Build history of the part. All positions in model axes, mm. Give positions to 0.01 mm unless a question says otherwise; leave off trailing zeros. Loops run counter-clockwise (first coordinate to the right, second up) from the corner with the lowest first, then second, coordinate; pieces in that order, holes last. Notation, with made-up numbers: (41.25, 75) -> (60.25, 75) arc R21 cw to (60.25, 103) -> close; hole circle Ø9 at (47.25, 71). An arc over 180 degrees is marked (long way). Answer as a JSON object with one key per item and string values. Group by question number.
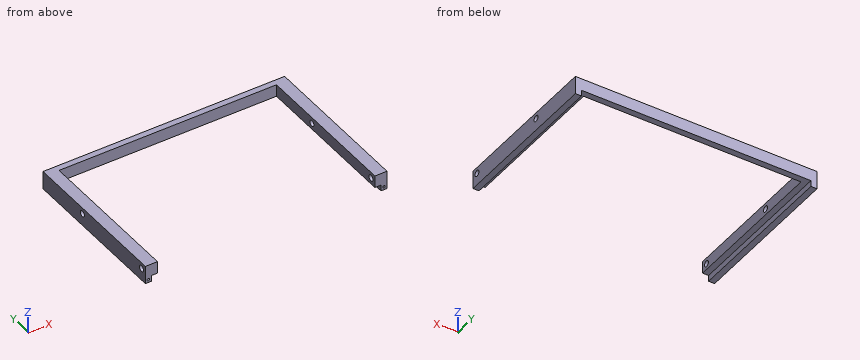
from build123d import *

# Parameters (mm, degrees)
F0_W      = 1300
F0_H      = 150
F1_DEPTH  = 50
F2_W      = 1300
F2_H      = 100
F3_DEPTH  = 50
F4_W      = 50
F4_H      = 100
F5_DEPTH  = 1800
F6_DEPTH  = 100
F7_W      = 100
F7_H      = 100
F8_DEPTH  = 1250
F9_W      = 50
F9_H      = 1300
F10_DEPTH = 50
F11_R     = 25
F12_DEPTH = 200
F13_R     = 25
F14_DEPTH = 200
F15_R     = 10
F16_DEPTH = 25
F17_R     = 10
F18_DEPTH = 25


with BuildPart() as f1:
    # F0 (on Right) → F1 (new body)
    with BuildSketch(Plane.YZ):
        Rectangle(F0_W, F0_H)
    extrude(amount=F1_DEPTH)

    # F2 (on face) → F3 (join)
    with BuildSketch(Plane.YZ.offset(50)):
        with Locations((0, 25)):
            Rectangle(F2_W, F2_H)
    extrude(amount=F3_DEPTH)

    # F4 (on face) → F5 (join)
    with BuildSketch(Plane.YZ.offset(100)):
        with Locations((625, 25)):
            Rectangle(F4_W, F4_H)
    extrude(amount=F5_DEPTH)

    # F6 (add): a face of the model
    f6_faces = [f1.faces().sort_by_distance(p)[0] for p in [
        (1900, 625, 25),
    ]]
    extrude(f6_faces, amount=F6_DEPTH)

    # F7 (on face) → F8 (join)
    with BuildSketch(Plane.XZ.offset(-600)):
        with Locations((1950, 25)):
            Rectangle(F7_W, F7_H)
    extrude(amount=F8_DEPTH)

    # F9 (on face) → F10 (join)
    with BuildSketch(Plane(origin=(0, 0, -25), x_dir=(1, 0, 0), z_dir=(0, 0, -1))):
        with Locations((1975, 0)):
            Rectangle(F9_W, F9_H)
    extrude(amount=F10_DEPTH)

    # F11 (on face) → F12 (cut)
    with BuildSketch(Plane.YZ.offset(100)):
        with Locations((150, 25)):
            Circle(F11_R)
        with Locations((-600, 25)):
            Circle(F11_R)
    extrude(amount=-F12_DEPTH, mode=Mode.SUBTRACT)

    # F13 (on face) → F14 (cut)
    with BuildSketch(Plane(origin=(1900, 0, 0), x_dir=(0, -1, 0), z_dir=(-1, 0, 0))):
        with Locations((-150, 25)):
            Circle(F13_R)
        with Locations((600, 25)):
            Circle(F13_R)
    extrude(amount=-F14_DEPTH, mode=Mode.SUBTRACT)

    # F15 (on face) → F16 (cut)
    with BuildSketch(Plane.XZ.offset(650)):
        with Locations((25, -50)):
            Circle(F15_R)
    extrude(amount=-F16_DEPTH, mode=Mode.SUBTRACT)

    # F17 (on face) → F18 (cut)
    with BuildSketch(Plane.XZ.offset(650)):
        with Locations((1975, -50)):
            Circle(F17_R)
    extrude(amount=-F18_DEPTH, mode=Mode.SUBTRACT)


solid = f1.part
(1) Saw through at C-C on z = 25. List the corners of the cut face in (x, y).
(2) Saw through at A-A on y = 258. List the corners of the cut face in (x, z).
(3) Pin check, flat tips, straight feed: pin 1 (16 mm diameter, centred on x = 25, z = -50, fed in from -Y); pin 2 (3 mm diameter, centred on x = 1384.5, z = -8, fed in from -Y). Stop position of each tip, or through.
(4) Probe line 1 along X through (y, z) = (509, 15.5); line 2 along X through (y, z) = (513, -61); line 3 along Z through (x, y) = (22, 150). List the from-to ranges inside material, lowest first. Write a range as [from, to].
(5) Saw through at B-B on y = -600. List the corners of the cut face in (x, z), plus the area to 3 significant figures.
(6) Saw through at D-D on x = 607. List the corners of the cut face in (y, z), plus the area to 3 significant figures.
Calculated:
{
 "1": {"outline": "(0, -650) -> (100, -650) -> (100, -625) -> (0, -625) -> close; (0, -575) -> (100, -575) -> (100, 125) -> (0, 125) -> close; (0, 175) -> (100, 175) -> (100, 600) -> (1900, 600) -> (1900, 175) -> (2000, 175) -> (2000, 650) -> (0, 650) -> close; (1900, -650) -> (2000, -650) -> (2000, -625) -> (1900, -625) -> close; (1900, -575) -> (2000, -575) -> (2000, 125) -> (1900, 125) -> close"},
 "2": {"outline": "(0, -75) -> (50, -75) -> (50, -25) -> (100, -25) -> (100, 75) -> (0, 75) -> close; (1900, -25) -> (1950, -25) -> (1950, -75) -> (2000, -75) -> (2000, 75) -> (1900, 75) -> close"},
 "3": {"pin 1": "stops at y = -625", "pin 2": "stops at y = 600"},
 "4": {"line 1": "x = [0, 100], [1900, 2000]", "line 2": "x = [0, 50], [1950, 2000]", "line 3": "z = [-75, 0], [50, 75]"},
 "5": {"outline": "(0, -75) -> (50, -75) -> (50, -25) -> (100, -25) -> (100, 0) -> (0, 0) -> close; (0, 50) -> (100, 50) -> (100, 75) -> (0, 75) -> close; (1900, -25) -> (1950, -25) -> (1950, -75) -> (2000, -75) -> (2000, 0) -> (1900, 0) -> close; (1900, 50) -> (2000, 50) -> (2000, 75) -> (1900, 75) -> close", "area": "15,000 mm^2"},
 "6": {"outline": "(600, -25) -> (650, -25) -> (650, 75) -> (600, 75) -> close", "area": "5,000 mm^2"}
}
